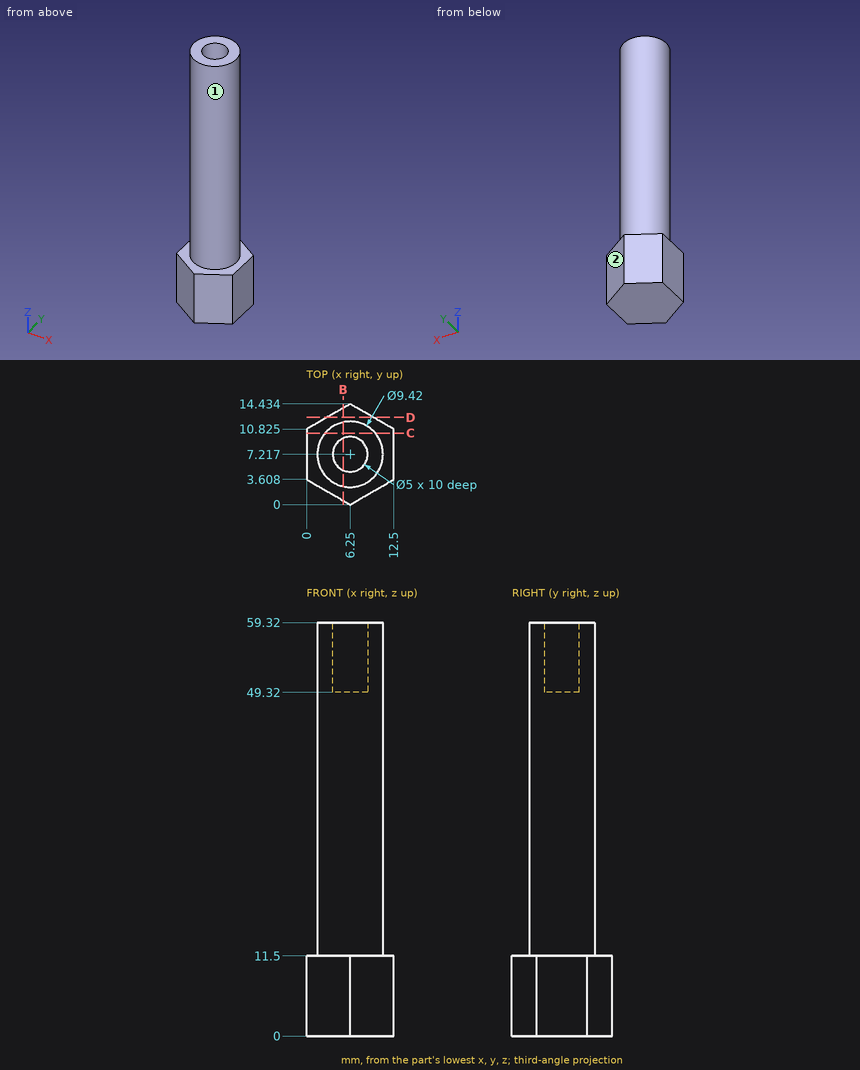
Source: three-view drawing plus pictorial views. Frame: mm from the lowest corner of the part. A direction names the side the tool comes from. Give positions to 0.01 mm unless a question says otherwise; leave off trailing zeros. Order: outer loops, then holes, each group sorted by start corner. A loop starts at its lowest first (then second) coordinate and runs counter-clockwise, first axis right, second up. Notation, with made-up numbers: M -21,40 L -13,40 A11 cw -13,51 Z; hole C 74.25,-5 d6. An arc over 180 degrees is marked long. Return JSON: item names as keys, results as strings.
Item 1: Access query for the marked faces 1 and 2. Directions: +Z, -Z, +X, -X, +Y, -Y. A direction counts if a zero-diameter tool reaches every point of the face in a straight line with its end or side. Return the directions, or none.
Solutions:
{"face 1": "+Z", "face 2": "+Z, -Z, +X, +Y"}
Item 2: First-contact query: P1, Ø6, axis at x = 10, z = 28.5, coming from the -Y side; P2, Ø1.5, axis at y = 5, z = 20.5, coming from the +X side (1 decimal); P3, Ø4, axis at x = 10, z = 21, coming from the -Y side (1 decimal). Flat tips, straight axial feed; report the tip coordinate or a pass-through.
Solutions:
{"P1": "y = 2.57", "P2": "x = 10.7", "P3": "y = 2.8"}
Item 3: Cut plane B-B (x = 5.25). Return loops of the section in (y, z) (1 decimal), then the cut area to 3 significant figures.
Solutions:
{"outline": "M 0.6,0 L 13.9,0 L 13.9,11.5 L 11.8,11.5 L 11.8,59.3 L 9.5,59.3 L 9.5,49.3 L 4.9,49.3 L 4.9,59.3 L 2.6,59.3 L 2.6,11.5 L 0.6,11.5 Z", "area": "547 mm^2"}
Item 4: Cut plane D-D (y = 12.5). Return loops of the section in (x, z).
Solutions:
{"outline": "M 2.9,0 L 9.6,0 L 9.6,11.5 L 2.9,11.5 Z"}
Item 5: Ray query, probe 1 along Y at (x, z) = (6.25, 56.5); probe 2 along Z at (x, y) = (9, 11.5); probe 3 along X at (y, z) = (8.5, 53) (1 decimal). Return the intervals inside material, ascending.
Solutions:
{"probe 1": "2.51 to 4.72, 9.72 to 11.93", "probe 2": "0 to 11.5", "probe 3": "1.7 to 4.1, 8.4 to 10.8"}
Item 6: Cut plane C-C (y = 10.25). Return loops of the section in (x, z).
Solutions:
{"outline": "M 0,0 L 12.5,0 L 12.5,11.5 L 9.85,11.5 L 9.85,59.32 L 2.65,59.32 L 2.65,11.5 L 0,11.5 Z"}
